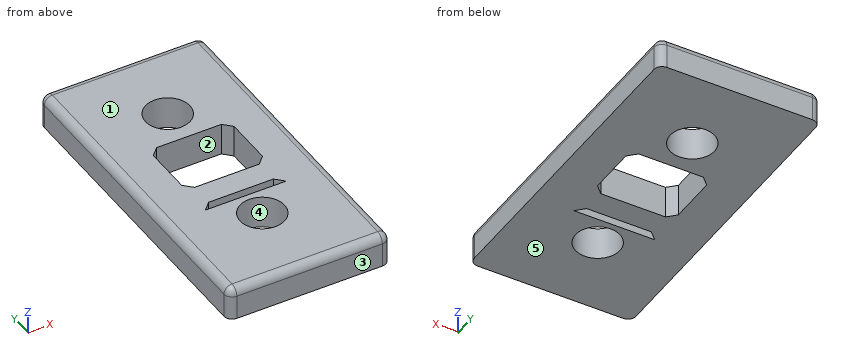
from build123d import *

# Parameters (mm, degrees)
F5_W     = 20
F5_H     = 40
F6_DEPTH = 4
F1_D     = 5.5
F2_R     = 1
F7_W     = 10
F7_H     = 1
F8_DEPTH = 25
F3_R     = 1
F4_SIZE  = 0.99999


# Not quite as in the source:
# - a fillet or chamfer is up to 0.001 mm smaller than in the source, because OpenCascade refuses the exact size
# - a feature names something its author has since deleted; it is built from what else it names


with BuildPart() as f6:
    # F5 (on Top) → F6 (new body)
    with BuildSketch(Plane.XY):
        Rectangle(F5_W, F5_H)
    extrude(amount=F6_DEPTH)

    # F1 (through all)
    with Locations(Plane.XY.offset(4)):
        with Locations((0, 10), (0, -10)):
            Hole(F1_D / 2)

    # F2
    f2_edges = [f6.edges().sort_by_distance(p)[0] for p in [
        (-10, -20, 2),
        (10, -20, 2),
        (-10, 20, 2),
        (10, 20, 2),
    ]]
    fillet(f2_edges, radius=F2_R)

    # F7 (on face) → F8 (cut)
    with BuildSketch(Plane.XY.offset(4)):
        Polygon((-5, -2.5), (5, -2.5), (5, 2.5), (5, 5.5), (-5, 5.5), (-5, 2.5), align=None)
        with Locations((0, -6)):
            Rectangle(F7_W, F7_H)
    extrude(amount=-F8_DEPTH, mode=Mode.SUBTRACT)

    # F3
    f3_edges = [f6.edges().sort_by_distance(p)[0] for p in [
        (0, -20, 4),
        (10, 0, 4),
        (0, 20, 4),
        (-10, 0, 4),
    ]]
    fillet(f3_edges, radius=F3_R)

    # F4 (size 1 in the source; OpenCascade refuses exactly that, so slightly less here)
    f4_edges = [f6.edges().sort_by_distance(p)[0] for p in [
        (-5, -5.5, 2),
        (5, -5.5, 2),
        (5, 5.5, 2),
        (-5, 5.5, 2),
        (-5, -2.5, 2),
        (5, -2.5, 2),
    ]]
    chamfer(f4_edges, length=F4_SIZE)


solid = f6.part
Check sheet for the modelled part. Datum: model origin and axes. Units: mm. Face numbers are marked on the shaded views. A direction names the side the tool comes from. Round coordinates to 2 decimals unless told otherwise and drop trailing zeros. Order: outer loops, then holes, each group sorted by start corner. A loop starts at its lowest first (then second) coordinate and runs counter-clockwise, first axis right, second up.
(1) Access from +Z, -Z, +X, -X, +Y, -Y to the whole of each face (thin tool, end or side, straight path). Record for the marked faces 1 and 2.
(2) Cross-section at C-C, the plane z = 1.6. State how many separate pieces and enclosed holes the cut face has, and give its area (3 significant figures).
(3) Go/stop test with a flat-tipped pin: P1, Ø4.5, axis at x = 0, y = -10, coming from the -Z side. Record where the tip stops, or that it passes through.
(4) Cross-section at A-A, the plane x = 0. Enter the section's corners in (y, z).
(5) Cross-section at D-D, the plane y = 3. Enter the section's corners in (x, z), and give its area (3 significant figures).
(6) Scan lines: probe 1 along Y at (x, z) = (0, 2.85); probe 2 along Y at (x, z) = (-3.75, 1.5); probe 3 along X at (y, z) = (3, 0.4). Record each from-to range of solid material in increasing order.
(7) Cross-section at B-B, the plane y = 10. Enter the section's corners in (x, z).
(8) Draft check along Y on the marked faces 3, 4 and 5. Enter one of: pulls with the +Y half, pulls with the -Y half, needs draft (parallel to the pull), parting line crosses it, or undercut.
Check sheet entries:
1. face 1: +Z, +X, -X, +Y, -Y
1. face 2: +Z, -Z
2. separate pieces: 1
2. enclosed holes: 4
2. area: 665 mm2
3. P1: passes through
4. outline: (-20, 0) - (-12.75, 0) - (-12.75, 4) - (-19, 4) arc R1 ccw to (-20, 3) - close; (-7.25, 0) - (-6.5, 0) - (-6.5, 4) - (-7.25, 4) - close; (-5.5, 0) - (-2.5, 0) - (-2.5, 4) - (-5.5, 4) - close; (5.5, 0) - (7.25, 0) - (7.25, 4) - (5.5, 4) - close; (12.75, 0) - (20, 0) - (20, 3) arc R1 ccw to (19, 4) - (12.75, 4) - close
5. outline: (-10, 0) - (-5, 0) - (-5, 4) - (-9, 4) arc R1 ccw to (-10, 3) - close; (5, 0) - (10, 0) - (10, 3) arc R1 ccw to (9, 4) - (5, 4) - close
5. area: 39.6 mm2
6. probe 1: y = -20 to -12.75, -7.25 to -6.5, -5.5 to -2.5, 5.5 to 7.25, 12.75 to 20
6. probe 2: y = -20 to -6.5, -5.5 to -2.5, 5.5 to 20
6. probe 3: x = -10 to -5, 5 to 10
7. outline: (-10, 0) - (-2.75, 0) - (-2.75, 4) - (-9, 4) arc R1 ccw to (-10, 3) - close; (2.75, 0) - (10, 0) - (10, 3) arc R1 ccw to (9, 4) - (2.75, 4) - close
8. face 3: pulls with the -Y half
8. face 4: undercut
8. face 5: needs draft
